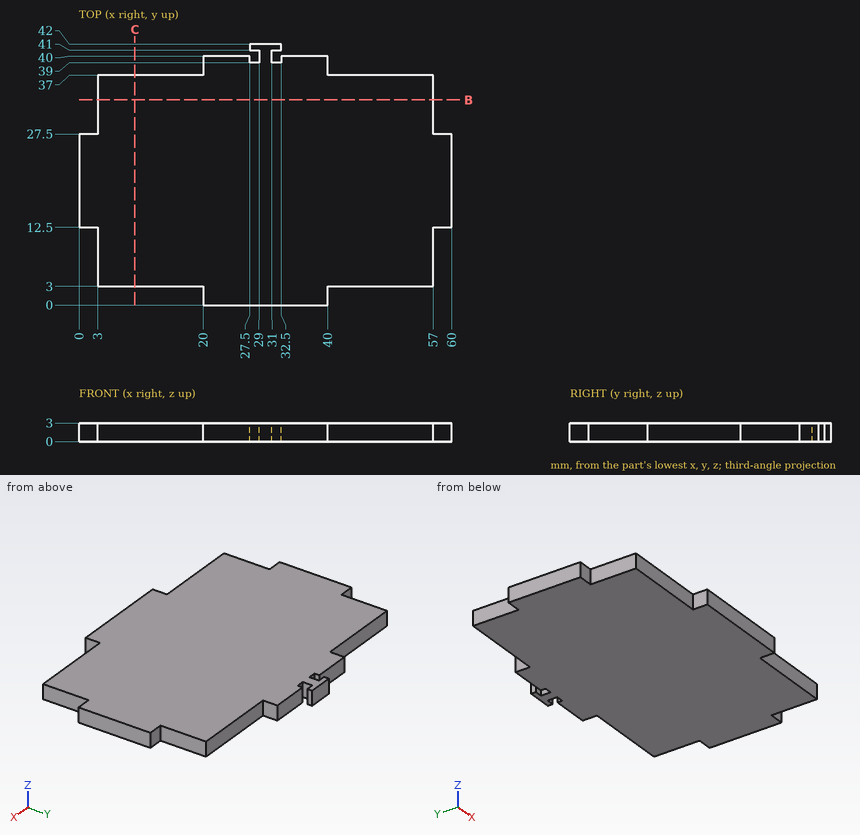
Design review of the part shown in the three views and the two pictorial views. Dimensions are in mm from the part's minimum x, y and z. Round coordinates to 2 decimals unless told otherwise and drop trailing zeros. Write each loop counter-clockwise with the first axis right and the second up, starting at its lowest first coordinate (ties: lowest second). Pieces come first, ordered by that corner, then holes. Notation, with made-up numbers: (17.25, -21) - (42.25, -21) arc R20 cw to (42.25, -10) - close; hole circle Ø9 at (75.5, -19.5). An arc over 180 degrees is marked (long way). Write item = value, one per line. Start each with the question number.
1. Consider section C-C on x = 9. State the section outline as (y, z) points, plus the area to 3 significant figures.
2. Consider section B-B on y = 33. State the section outline as (x, z) points.
3. Wall thickness on L1, parallel to X at y = 39.5, z = 1.15; L2, parallel to X at y = 35.5, z = 1.7; L3, parallel to Y at x = 8, z = 2.85: over which ranges is each line inside the solid? List them lowest first.
4. For pin 1 Ø0.9 at (x, z) = (59, 2) entering from +Y; pin 2 Ø0.5 at (y, z) = (41.5, 1) entering from -X; pin 3 Ø0.9 at (x, z) = (2, 2) entering from -Y; pin 4 Ø8 at (x, y) = (47, 36.5) entering from -Z, all flat-tipped, find the tip position at first contact; note any pin that passes through.
Evaluation:
q1.outline = (3, 0) - (37, 0) - (37, 3) - (3, 3) - close
q1.area = 102 mm2
q2.outline = (3, 0) - (57, 0) - (57, 3) - (3, 3) - close
q3.L1 = 20 to 27.5, 29 to 31, 32.5 to 40
q3.L2 = 3 to 57
q3.L3 = 3 to 37
q4.pin_1 = 27.5
q4.pin_2 = 27.5
q4.pin_3 = 12.5
q4.pin_4 = 0
